The listing builds one solid part. Answer for the finished solid, in the listing's coordinates (mm). A direction names the side the tool comes from. Give positions to 0.01 mm unless a question says otherwise; leave off trailing zeros. Write each loop counter-clockwise with the first axis right and the second up, starting at its lowest first coordinate (ties: lowest second). Pieces come first, ordered by that corner, then holes. Notation, with made-up numbers: (86, -2) - (132, -2) arc R29 ccw to (132, 23) - close; hole circle Ø3 at (49.25, 3). An arc over 180 degrees is marked (long way). Answer as CSV lines item,"result". Start each with the question number.
(1) Find section D-D (y = -35.5). Write down the section's boundary in (x, z), then the cut area to 3 significant figures.
(2) For a pull along Y with two mould halves and no side action, classify faces 1 (the face through (22.535, -13.453, 10.162)), 2 (the face through (22, -17.055, 5)), 3 (the face through (0.042, 11.503, -20.356)) as pulls with the +Y half, pulls with the -Y half, needs draft (parallel to the pull), parting line crosses it, or undercut.
(3) Find section A-A (x = 11.5). Write down the section's boundary in (y, z).
(4) Each of these flat-tipped pins is pushed along its axis until it touches: pin 1 Ø1.5 at (x, z) = (23.5, 4) entering from -Y (3 decimals); pin 2 Ø4 at (x, y) = (-23.5, -39.5) entering from +Z; pin 3 Ø1 at (x, y) = (19, -46.5) entering from +Z. Where does it stop, or does it pass through?
(5) For faces 4 (the face through (-22, -17.055, 5)), 5 (the face through (0, -83.012, -13)), 6 (the face through (0, 22, -5)), 7 (the face through (-11, 0, 6)), determine the directions among +Z, -Z, +X, -X, +Y, -Y from which every point of the face is accessible in a straight line to the end or side of a thin tool.
(6) Straight lines are drawn through the part: probe 1 along X at (y, z) = (-100, 5); probe 2 along Y at (x, z) = (-18, -6); probe 3 along Z at (x, y) = (0.75, 32.5). For each, find the intervals that lie inside material, in ascending order.
(7) Find section B-B (y = 32.5). Write down the section's boundary in (x, z), then the cut area to 3 significant figures.
(8) Find section C-C (z = 9.5). Write down the section's boundary in (x, y).
from build123d import *

# Parameters (mm, degrees)
F1_DEPTH      = 20
F1_DEPTH_BACK = 20
F2_DEPTH      = 25
F2_DEPTH_BACK = 25
F3_DEPTH      = 3
F3_DEPTH_BACK = 3
F0_R          = 11.25
F4_DEPTH      = 3
F5_T1_DEPTH   = 79.3350946098
F5_T3_DEPTH   = 53.4182341985
F5_T5_DEPTH   = 77.6393497362
F5_T7_DEPTH   = 53.8076131524
F5_T9_DEPTH   = 40.7011174437
F5_T11_DEPTH  = 34.8143073008


# Not quite as in the source:
# - a fillet or chamfer that OpenCascade refuses, or shapes differently, is made with other operations: its cross-section is extruded or revolved along the edge and cut away or added


with BuildPart() as f1:
    # F0 (on Right) → F1 (new body, two sides)
    with BuildSketch(Plane.YZ) as f1_sk:
        Polygon((0, 0), (0, 26.4743264821), (-15.4693145305, 49.9219790902), (-66.8067783117, 42.1494067516), (-109.735481441, 10.023953287), (-109.735481441, 0), (-83.011649549, 0), (-17.0549713075, 0), (-17.0549713075, 12.6967383549), (-7.9574938864, 12.6967383549), align=None)
    extrude(amount=F1_DEPTH)
    extrude(f1_sk.sketch, amount=-F1_DEPTH_BACK)

    # F0 (on Right) → F2 (join, two sides)
    with BuildSketch(Plane.YZ) as f2_sk:
        Polygon((-29.8482906073, -33.9278131723), (-6.5574786317, -18.399150059), (0, -14.0270879492), (0, 0), (-7.9574938864, 12.6967383549), (-17.0549713075, 12.6967383549), (-17.0549713075, 0), (-83.011649549, 0), (-83.011649549, -26.5361145139), align=None)
    extrude(amount=F2_DEPTH)
    extrude(f2_sk.sketch, amount=-F2_DEPTH_BACK)

    # F0 (on Right) → F3 (join, two sides)
    with BuildSketch(Plane.YZ) as f3_sk:
        with BuildLine():
            ThreePointArc((30.0759126991, -22.3690366524), (10.142147556, 2.5251602116), (35.1261815426, 22.346211547))
            Line((35.1261815426, 22.346211547), (0, 26.4743264821))
            Line((0, 26.4743264821), (0, 0))
            Line((0, 0), (0, -14.0270879492))
            Line((0, -14.0270879492), (-6.5574786317, -18.399150059))
            Line((-6.5574786317, -18.399150059), (30.0759126991, -22.3690366524))
        make_face()
    extrude(amount=F3_DEPTH)
    extrude(f3_sk.sketch, amount=-F3_DEPTH_BACK)

    # F0 (on Right) → F4 (join)
    with BuildSketch(Plane.YZ):
        with BuildLine():
            ThreePointArc((30.0759126991, -22.3690366524), (47.5284403005, -16.7450285797), (55, 0))
            ThreePointArc((55, 0), (49.3127791383, 14.9526070518), (35.1261815426, 22.346211547))
            ThreePointArc((35.1261815426, 22.346211547), (10.142147556, 2.5251602116), (30.0759126991, -22.3690366524))
        make_face()
        with Locations((32.5, 0)):
            Circle(F0_R, mode=Mode.SUBTRACT)
    extrude(amount=F4_DEPTH)

    # F5: chamfer of 5 on 11 edges, made by hand

    # F5_s2 → F5_t1 (cut)
    with BuildSketch(Plane(origin=(0, -12.3102659146, -9.2123182381), x_dir=(1, 0, 0), z_dir=(0, -0.8006358159, -0.5991513084))):
        Polygon((20, 68.7736932965), (15, 73.7736932965), (20, 73.7736932965), align=None)
        Polygon((-20, 68.7736932965), (-15, 73.7736932965), (-20, 73.7736932965), align=None)
    extrude(amount=F5_T1_DEPTH, mode=Mode.SUBTRACT)

    # F5_s4 → F5_t3 (cut)
    with BuildSketch(Plane.YZ.offset(-26.7091170992)):
        Polygon((-107.7312379828, 11.5238176028), (-109.735481441, 7.5206385233), (-109.735481441, 10.023953287), align=None)
    extrude(amount=F5_T3_DEPTH, mode=Mode.SUBTRACT)

    # F5_s6 → F5_t5 (cut)
    with BuildSketch(Plane(origin=(0, 4.9797561094, 0.7539428662), x_dir=(1, 0, 0), z_dir=(0, -0.9887321325, -0.1496955918))):
        Polygon((20, 46.675153037), (15, 51.675153037), (20, 51.675153037), align=None)
        Polygon((-15, 51.675153037), (-20, 46.675153037), (-20, 51.675153037), align=None)
    extrude(amount=F5_T5_DEPTH, mode=Mode.SUBTRACT)

    # F5_s8 → F5_t7 (cut)
    with BuildSketch(Plane(origin=(0, -5.0883568573, 7.7126897705), x_dir=(1, 0, 0), z_dir=(0, -0.5506900388, 0.8347098185))):
        Polygon((15, 14.5791478777), (20, 9.5791478777), (20, 14.5791478777), align=None)
        Polygon((-15, 14.5791478777), (-20, 9.5791478777), (-20, 14.5791478777), align=None)
    extrude(amount=F5_T7_DEPTH, mode=Mode.SUBTRACT)

    # F5_s10 → F5_t9 (cut)
    with BuildSketch(Plane(origin=(0, 6.8285367479, -10.8954082369), x_dir=(1, 0, 0), z_dir=(0, -0.5310558712, 0.8473368053))):
        Polygon((20, 0), (25, -5), (25, 0), align=None)
        Polygon((-25, -5), (-20, 0), (-25, 0), align=None)
    extrude(amount=F5_T9_DEPTH, mode=Mode.SUBTRACT)

    # F5_s12 → F5_t11 (cut)
    with BuildSketch(Plane.XZ.offset(-4.9009210535)):
        Polygon((25, 7.6967383549), (20, 12.6967383549), (25, 12.6967383549), align=None)
        Polygon((-25, 7.6967383549), (-20, 12.6967383549), (-25, 12.6967383549), align=None)
    extrude(amount=F5_T11_DEPTH, mode=Mode.SUBTRACT)


solid = f1.part
Result set:
1,outline,"(-25, -33.14) - (25, -33.14) - (25, 0) - (20, 0) - (20, 41.83) - (15, 46.89) - (-15, 46.89) - (-20, 41.83) - (-20, 0) - (-25, 0) - close"
1,area,"3,510 mm^2"
2,face 1,"needs draft"
2,face 2,"pulls with the -Y half"
2,face 3,"undercut"
3,outline,"(-109.74, 0) - (-83.01, 0) - (-83.01, -26.54) - (-29.85, -33.93) - (0, -14.03) - (0, 26.47) - (-15.47, 49.92) - (-66.81, 42.15) - (-107.73, 11.52) - (-109.74, 7.52) - close"
4,pin 1,"y = -17.055"
4,pin 2,"z = 0"
4,pin 3,"z = 41.69"
5,face 4,"+Z, -X, -Y"
5,face 5,"-Z, +X, -X, -Y"
5,face 6,"-X, +Y"
5,face 7,"+Z, -Z, -X, +Y"
6,probe 1,"-20 to 20"
6,probe 2,"-83.01 to 0"
6,probe 3,"-22.5 to -11.25, 11.25 to 22.65"
7,outline,"(-3, 22.5) - (0, 22.5) - (0, 11.25) - (3, 11.25) - (3, 22.65) - (-3, 22.65) - close; (0, -22.5) - (3, -22.5) - (3, -11.25) - (0, -11.25) - close"
7,area,"68.4 mm^2"
8,outline,"(-23.2, -17.05) - (-20, -17.05) - (-20, -102.09) - (-16.01, -108.74) - (16.01, -108.74) - (20, -102.09) - (20, -17.05) - (23.2, -17.05) - (23.2, -9.73) - (20, -5.95) - (20, 0) - (3, 0) - (3, 26.47) - (0, 26.47) - (0, 12.1) - (-3, 12.1) - (-3, 0) - (-20, 0) - (-20, -5.95) - (-23.2, -9.73) - close; (0, 38.53) - (3, 38.53) - (3, 52.9) - (0, 52.9) - close"
